from build123d import *

# Parameters (mm, degrees)
SKETCH1_R           = 6.35
BOSS_EXTRUDE1_DEPTH = 22.86
CHAMFER1_SIZE       = 2.54
SKETCH2_R           = 1.9812
CUT_EXTRUDE1_DEPTH  = 14.2748


with BuildPart() as part:
    # Sketch1 → Boss-Extrude1 (new, symmetric)
    with BuildSketch(Plane.XY):
        Circle(SKETCH1_R)
    extrude(amount=BOSS_EXTRUDE1_DEPTH, both=True)

    # Chamfer1
    chamfer1_edges = [part.edges().sort_by_distance(p)[0] for p in [
        (-6.35, 0, 22.86),
    ]]
    chamfer(chamfer1_edges, length=CHAMFER1_SIZE)

    # Sketch2 → Cut-Extrude1 (cut)
    with BuildSketch(Plane(origin=(0, 0, -22.86), x_dir=(-1, 0, 0), z_dir=(0, 0, -1))):
        Circle(SKETCH2_R)
    extrude(amount=-CUT_EXTRUDE1_DEPTH, mode=Mode.SUBTRACT)


solid = part.part
Could you check a few things on this model? Use its own coordinates, in mm. A direction names the side the tool comes from. Coordinates: 2 decimals unless noted, no trailing zeros. Order: outer loops, then holes, each group sorted by start corner. A loop starts at its lowest first (then second) coordinate and runs counter-clockwise, first axis right, second up. Notation, with made-up numbers: (32, 87.25) -> (56, 87.25) arc R10 cw to (56, 94.25) -> close; hole circle Ø4 at (69, -14). An arc over 180 degrees is marked (long way). One line per question, with ' | ' between items.
Q1. If I drill on L1, parallel to Y at x = 0, z = -12; L2, parallel to Z at x = -0.5, y = -0.5; L3, parallel to X at y = 0.5, z = -14, over which ranges is the centre line in solid material (lowest first)?
Return value:
L1: -6.35 to -1.98, 1.98 to 6.35 | L2: -8.59 to 22.86 | L3: -6.33 to -1.92, 1.92 to 6.33
Q2. Imagine slicing it at A-A on x = 0. Please give me the cut outline in (y, z), and give its area (3 significant figures).
Return value:
outline: (-6.35, -22.86) -> (-1.98, -22.86) -> (-1.98, -8.59) -> (1.98, -8.59) -> (1.98, -22.86) -> (6.35, -22.86) -> (6.35, 20.32) -> (3.81, 22.86) -> (-3.81, 22.86) -> (-6.35, 20.32) -> close | area: 518 mm²
Q3. Thinking about a two-plate mould opening in Y: for faces 3 (the face through (1, 2, -22.86)), 4 (the face through (0, 0, -8.585)), 5 (the face through (-1.38, -6.2, -0.97)), which applies, pulls with the +Y half, pulls with the -Y half, needs draft (parallel to the pull), parting line crosses it, or undercut?
Return value:
face 3: needs draft | face 4: undercut | face 5: parting line crosses it
Q4. I'm going to push flat-ended pins straight in: P1, Ø5, axis at y = -4, z = -13, coming from the +X side; P2, Ø2, axis at x = -0.5, y = -0.5, coming from the -Z side; P3, Ø1, axis at y = 5, z = -2, coming from the +X side. Where does each tip first touch, or does it pass through?
Return value:
P1: x = 6.17 | P2: z = -8.59 | P3: x = 4.48
Q5. On a 3-axis mill with a long thin cutter (end or side, diameter ignored), from which of +Z, -Z, +X, -X, +Y, -Y can I reach the whole of each face in a straight line? I mean faces 1 (the face through (0.258, 1.964, -15.823)), 2 (the face through (0, 0, 22.86)). Say none if no direction works.
Return value:
face 1: -Z | face 2: +Z, +X, -X, +Y, -Y
Q6. Imagine slicing it at B-B on z = 8. Please give me the cut outline in (x, y).
Return value:
outline: circle Ø12.7 at (0, 0)
